Can you work these out from the model? Positions are in its coordinate system, mm. Face numbers are marked on the shaded views. A direction names the side the tool comes from. Coordinates: 2 decimals unless noted, no trailing zeros. Loops run counter-clockwise (first coordinate to the right, second up) from the corner with the lowest first, then second, coordinate; pieces in that order, holes last. Notation, with made-up numbers: (50.5, 45) -> (87.5, 45) arc R20 ccw to (87.5, 83) -> close; hole circle Ø7 at (58, 30.5). An arc over 180 degrees is marked (long way). Use one line per item in the form item = value. Start each with the question number.
(1) On a 3-axis mill with a long thin cutter (end or side, diameter ignored), from which of +Z, -Z, +X, -X, +Y, -Y can I reach the whole of each face in a straight line? I mean the marked faces 1 and 2. Say none if no direction works.
(2) Imagine slicing it at B-B (y = 4). List the corners of the cut face in (x, z) for me.
(3) Imagine slicing it at D-D (z = -12). List the corners of the cut face in (x, y) for me, plus the area to 3 significant figures.
(4) Imagine slicing it at A-A (z = -4). List the corners of the cut face in (x, y) for me, plus the area to 3 significant figures.
(5) I'm going to push flat-ended pins straight in: pin 1 (12 mm diameter, centred on y = 18, z = -34.5, fed in from -X); pin 2 (3 mm diameter, centred on x = 4, y = 4, fed in from -Z); pin 3 (3.5 mm diameter, centred on x = 4, y = 21.5, fed in from +Z); pin 4 (0.8 mm diameter, centred on x = 3.5, z = -12, fed in from +Y). Where does each tip first touch, or does it pass through?
(6) Imagine slicing it at C-C (x = 1.75). State how many separate pieces and enclosed holes the cut face has, plus the area to 3 significant figures.
(7) Thinking about a two-plate mould opening in Y: for the marked faces 3, 4, 5 and 6, which applies, released by +Y, released by -Y, zero draft, split by the parting line, or undercut?
(8) I need wall thicknesses on line 1 (Y direction, x = 4, z = -2.5); line 2 (Y direction, x = 5, z = -6); line 3 (Y direction, x = 7, z = -5). Which ranges of each line are inside material? Lowest first, please. Write a range as [from, to].
```python
from build123d import *
from build123d.topology import SkipClean

# Parameters (mm, degrees)
SKETCH1_R           = 1.55
BOSS_EXTRUDE1_DEPTH = 8
SKETCH2_R           = 3.2
CUT_EXTRUDE1_DEPTH  = 1.5
CUT_EXTRUDE1_DRAFT  = -60
BOSS_EXTRUDE2_START = 0.75
SKETCH3_R           = 2.5
SKETCH3_R_2         = 1.55
BOSS_EXTRUDE2_DEPTH = 0.75
SKETCH4_R           = 1.55
CUT_EXTRUDE2_DEPTH  = 20
SKETCH5_W           = 2.6
SKETCH5_H           = 5.7
CUT_EXTRUDE3_DEPTH  = 60.371710435
FILLET2_R           = 1.5
FILLET3_R           = 5
FILLET4_R           = 10
CHAMFER1_SIZE       = 0.5


with BuildPart() as part:
    # Sketch1 → Boss-Extrude1 (new body)
    with BuildSketch(Plane(origin=(0, 0, 0), x_dir=(0, 0, -1), z_dir=(1, 0, 0))):
        Polygon((0, 0), (50, 0), (50, 31), (35, 31), (35, 25.5), (0, 25.5), (0, 17.5), (35, 17.5), (35, 8), (0, 8), align=None)
        with Locations((42.5, 23.25)):
            Circle(SKETCH1_R, mode=Mode.SUBTRACT)
    extrude(amount=BOSS_EXTRUDE1_DEPTH)


with BuildPart() as cut_extrude1_tool:
    # Sketch2 → Cut-Extrude1 (with draft: the straight prism first)
    with BuildSketch(Plane(origin=(8, 0, 0), x_dir=(0, 0, -1), z_dir=(1, 0, 0))):
        with Locations((42.5, 23.25)):
            Circle(SKETCH2_R)
    extrude(amount=-CUT_EXTRUDE1_DEPTH)
    # Cut-Extrude1: the draft: its side faces are tilted about the plane it starts from
    cut_extrude1_sides = [cut_extrude1_tool.faces().sort_by_distance(p)[0] for p in [
        (7.25, 23.25, -39.3),
    ]]
    draft(cut_extrude1_sides, Plane(origin=(8, 0, 0), x_dir=(0, 0, -1), z_dir=(1, 0, 0)), CUT_EXTRUDE1_DRAFT)


with BuildPart() as part_1:
    add(part.part)

    # Cut-Extrude1: cut by cut_extrude1_tool
    add(cut_extrude1_tool.part, mode=Mode.SUBTRACT)

    # Sketch3 → Boss-Extrude2 (add)
    with SkipClean():  # the faces are left unmerged after this step: merging them gives an invalid solid
        with BuildSketch(Plane.ZY.offset(BOSS_EXTRUDE2_START)):
            with Locations(Location((-42.5, 23.25, 0), (0, 0, 180))):
                Circle(SKETCH3_R)
            with Locations((-42.5, 23.25)):
                Circle(SKETCH3_R_2, mode=Mode.SUBTRACT)
        extrude(amount=-BOSS_EXTRUDE2_DEPTH)

    # Sketch4 → Cut-Extrude2 (cut)
    with SkipClean():  # the faces are left unmerged after this step: merging them gives an invalid solid
        with BuildSketch(Plane.XY):
            with Locations((4, 21.5)):
                Circle(SKETCH4_R)
            with Locations((4, 4)):
                Circle(SKETCH4_R)
        extrude(amount=-CUT_EXTRUDE2_DEPTH, mode=Mode.SUBTRACT)

    # Sketch5 → Cut-Extrude3 (cut, through all)
    with SkipClean():  # the faces are left unmerged after this step: merging them gives an invalid solid
        with BuildSketch(Plane.ZY):
            with Locations((-12, 21.5)):
                Rectangle(SKETCH5_W, SKETCH5_H)
            with Locations((-12, 4)):
                Rectangle(SKETCH5_W, SKETCH5_H)
        extrude(amount=-CUT_EXTRUDE3_DEPTH, mode=Mode.SUBTRACT)

    # Fillet2
    fillet2_edges = [part_1.edges().sort_by_distance(p)[0] for p in [
        (4, 8, -35),
        (4, 17.5, -35),
        (4, 25.5, -35),
        (4, 31, -35),
    ]]
    fillet(fillet2_edges, radius=FILLET2_R)

    # Fillet3
    fillet3_edges = [part_1.edges().sort_by_distance(p)[0] for p in [
        (4, 31, -50),
    ]]
    fillet(fillet3_edges, radius=FILLET3_R)

    # Fillet4
    fillet4_edges = [part_1.edges().sort_by_distance(p)[0] for p in [
        (4, 0, -50),
    ]]
    fillet(fillet4_edges, radius=FILLET4_R)

    # Chamfer1
    chamfer1_edges = [part_1.edges().sort_by_distance(p)[0] for p in [
        (0, 21.5, 0),
        (0, 4, 0),
        (4, 8, 0),
        (4, 17.5, 0),
        (4, 25.5, 0),
        (4, 0, 0),
        (8, 21.5, 0),
        (8, 4, 0),
    ]]
    chamfer(chamfer1_edges, length=CHAMFER1_SIZE)


solid = part_1.part
```
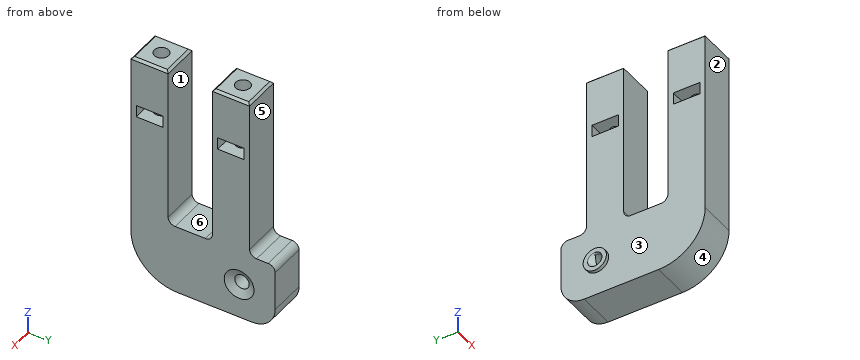
Worked out:
q1.face_1 = +Z, +X, -X
q1.face_2 = +Z, -Z, +X, -X, -Y
q2.outline = (0, -48) -> (8, -48) -> (8, -13.3) -> (5.55, -13.3) -> (5.55, -20) -> (2.45, -20) -> (2.45, -13.3) -> (0, -13.3) -> close; (0, -10.7) -> (2.45, -10.7) -> (2.45, 0) -> (0.5, 0) -> (0, -0.5) -> close; (5.55, -10.7) -> (8, -10.7) -> (8, -0.5) -> (7.5, 0) -> (5.55, 0) -> close
q3.outline = (0, 0) -> (8, 0) -> (8, 1.15) -> (0, 1.15) -> close; (0, 6.85) -> (8, 6.85) -> (8, 8) -> (0, 8) -> close; (0, 17.5) -> (8, 17.5) -> (8, 18.65) -> (0, 18.65) -> close; (0, 24.35) -> (8, 24.35) -> (8, 25.5) -> (0, 25.5) -> close
q3.area = 36.8 mm2
q4.outline = (0, 0) -> (8, 0) -> (8, 8) -> (0, 8) -> close; (0, 17.5) -> (8, 17.5) -> (8, 25.5) -> (0, 25.5) -> close; hole circle Ø3.1 at (4, 4); hole circle Ø3.1 at (4, 21.5)
q4.area = 113 mm2
q5.pin_1 = 0
q5.pin_2 = -48.93
q5.pin_3 = 0
q5.pin_4 = 25.5
q6.separate_pieces = 1
q6.enclosed_holes = 3
q6.area = 961 mm2
q7.face_3 = zero draft
q7.face_4 = released by -Y
q7.face_5 = released by +Y
q7.face_6 = undercut
q8.line_1 = [0, 2.45], [5.55, 8], [17.5, 19.95], [23.05, 25.5]
q8.line_2 = [0, 2.82], [5.18, 8], [17.5, 20.32], [22.68, 25.5]
q8.line_3 = [0, 8], [17.5, 25.5]
